CAD build for the part. Positions are in the model's coordinates, mm. Give positions to 0.01 mm unless a question says otherwise; leave off trailing zeros. Loops run counter-clockwise (first coordinate to the right, second up) from the corner with the lowest first, then second, coordinate; pieces in that order, holes last. Notation, with made-up numbers: M -25,-2.5 L 33,-2.5 A26 cw 33,13.5 Z; hole C -10.75,-10 d4. An arc over 180 degrees is marked long. Answer as CSV lines item,"result".
Autodesk Inventor part; units mm, degrees
ref_plane "YZ Plane" through (0, 0, 0) normal (1, 0, 0) x (0, 1, 0)
ref_plane "XZ Plane" through (0, 0, 0) normal (0, 1, 0) x (-1, 0, 0)
ref_plane "XY Plane" through (0, 0, 0) normal (0, 0, 1) x (1, 0, 0)
sketch "Sketch1" plane through (0, 0, 0) normal (1, 0, 0) x (0, 1, 0)
  circle A0 centre (0, 0) radius 10
  circle A1 centre (0, 0) radius 20
  dimension "d0" = 20
  dimension "d3" = 40
extrude "Extrusion1" add sketch "Sketch1" along normal blind 4
sketch "Sketch3" plane through (4, 0, 0) normal (1, 0, 0) x (0, 0, -1)
  line L0 (0, 0) -> (15.75, 0)
  circle A0 centre (15.75, 0) radius 2.5
  dimension "d4" = 15.75
  dimension "d5" = 5
extrude "Extrusion2" cut sketch "Sketch3" against normal blind 4
pattern_circular "Circular Pattern1" count 4 over 360 about axis through (-10, 0, 0) along (1, 0, 0) of "Extrusion2"
sketch "Sketch4" plane through (4, 0, 0) normal (1, 0, 0) x (0, 0, -1)
  line L0 (0, 0) -> (11.1369, 11.1369)
  line L1 (0, 0) -> (15.75, 0) construction
  circle A0 centre (11.1369, 11.1369) radius 2.5
  dimension "d11" = 15.75
  dimension "d12" = 45
  dimension "d13" = 5
extrude "Extrusion3" cut sketch "Sketch4" against normal blind 4
thread "Thread1"
pattern_circular "Circular Pattern2" count 4 over 360 about axis through (-10, 0, 0) along (1, 0, 0) of "Extrusion3"
properties part number "Robot Flange"
Q1. Cut at D-D (y = -15.75). Write the cut outline in (x, z), and give its area (3 significant figures).
Solution:
outline,"M 0,-12.33 L 4,-12.33 L 4,-2.5 L 0,-2.5 Z; M 0,2.5 L 4,2.5 L 4,12.33 L 0,12.33 Z"
area,"78.6 mm²"
Q2. Cut at A-A (y = 0). Write the cut outline in (x, z), and give its area (3 significant figures).
Solution:
outline,"M 0,-20 L 4,-20 L 4,-18.25 L 0,-18.25 Z; M 0,-13.25 L 4,-13.25 L 4,-10 L 0,-10 Z; M 0,10 L 4,10 L 4,13.25 L 0,13.25 Z; M 0,18.25 L 4,18.25 L 4,20 L 0,20 Z"
area,"40.0 mm²"
Q3. Wall check: line 1 (Z direction, x = 2.45, y = 0); line 2 (Y direction, x = 3.4, z = 1.5); line 3 (Z direction, x = 2.9, y = 11.5). Give the ranges that are in metal, low to high. Write a range as [from, to].
Solution:
line 1,"z = [-20, -18.25], [-13.25, -10], [10, 13.25], [18.25, 20]"
line 2,"y = [-19.94, -17.75], [-13.75, -9.89], [9.89, 13.75], [17.75, 19.94]"
line 3,"z = [-16.36, -13.61], [-8.66, 8.66], [13.61, 16.36]"
Q4. Pin check, flat tips, straight feed: P1, Ø3, axis at y = 11.14, z = 11.14, coming from the -X side; P2, Ø1.5, axis at x = 3, z = -4.5, coming from the -Y side; P3, Ø1, axis at x = 3.5, z = -7.5, coming from the -Y side (3 decimals); P4, Ø1.5, axis at x = 1, z = -9, coming from the -Y side. Stop position of each tip, or through.
Solution:
P1,"passes through"
P2,"stops at y = -19.65"
P3,"stops at y = -18.735"
P4,"stops at y = -18.22"
Q5. Mould opens along Y. For faces 1 (the cylindrical face through (1.972, -4.336, 19.524)), 2 (the cylindrical face through (2.028, 13.252, 0.11)), 3 (the flat face through (4, -5, 9)) say: released by +Y, released by -Y, zero draft, split by the parting line, or undercut.
Solution:
face 1,"split by the parting line"
face 2,"undercut"
face 3,"zero draft"
Q6. Cut at C-C (x = 0.7). Give the number of separate pieces and of enclosed holes in the cut face, and give its area (3 significant figures).
Solution:
separate pieces,"1"
enclosed holes,"9"
area,"785 mm²"
